Geometry: final body of the model. Coordinates: model frame, mm. Round coordinates to 2 decimals unless told otherwise and drop trailing zeros. Order: outer loops, then holes, each group sorted by start corner. A loop starts at its lowest first (then second) coordinate and runs counter-clockwise, first axis right, second up. Notation, with made-up numbers: M 70,44.5 L 112,44.5 A30 cw 112,72.5 Z; hole C 82.25,38 d10. An arc over 180 degrees is marked long. Return JSON: item names as keys, results as strings. Group by question number.
Q1. Contact query for flat-ended pins moving along their axis: pin 1 (5 mm diameter, centred on x = -5, y = -8, fed in from +Z); pin 2 (10 mm diameter, centred on x = 0, z = -6, fed in from -Y); pin 3 (1.1 mm diameter, centred on y = 3, z = 59, fed in from +X). Output: stop coordinate, or through.
Q2. Cut plane A-A on x = 5. Output: boundary loops of the cut face in (y, z), and give its area (3 significant figures).
Q3. Cut plane C-C on z = -23.5. Output: boundary loops of the cut face in (x, y).
Q4. Ray query, probe 1 along Y at (x, z) = (3.5, -9); probe 2 along Z at (x, y) = (8, -3); probe 3 along Z at (x, y) = (-9.5, 3). Return the intervals inside material, ascending.
Q5. Cut plane B-B on y = -7.5. Output: boundary loops of the cut face in (x, z).
```python
from build123d import *

# Parameters (mm, degrees)
SKETCH1_W           = 36
SKETCH1_H           = 1
BOSS_EXTRUDE1_DEPTH = 65
BOSS_EXTRUDE2_DEPTH = 5
SKETCH3_W           = 36
SKETCH3_H           = 2
BOSS_EXTRUDE3_DEPTH = 10
CUT_EXTRUDE1_REACH  = 76.334


with BuildPart() as part:
    # Sketch1 → Boss-Extrude1 (new, symmetric)
    with BuildSketch(Plane.XY):
        Rectangle(SKETCH1_W, SKETCH1_H)
    extrude(amount=BOSS_EXTRUDE1_DEPTH, both=True)

    # Sketch2 → Boss-Extrude2 (add, symmetric)
    with BuildSketch(Plane.XY.offset(60)):
        Polygon((-15, 0.5), (-15, 2.5), (-16.5, 2.5), (-16.5, 3.5), (16.5, 3.5), (16.5, 2.5), (15, 2.5), (15, 0.5), align=None)
    extrude(amount=BOSS_EXTRUDE2_DEPTH, both=True)

    # Sketch3 → Boss-Extrude3 (add)
    with BuildSketch(Plane.XZ.offset(0.5)):
        with Locations((0, -54)):
            Rectangle(SKETCH3_W, SKETCH3_H)
    extrude(amount=BOSS_EXTRUDE3_DEPTH)

    # Sketch4 → Cut-Extrude1 (cut, up to next)
    with BuildSketch(Plane(origin=(16.5, 0, 0), x_dir=(0, 0, -1), z_dir=(1, 0, 0)), mode=Mode.PRIVATE) as cut_extrude1_sk1:
        Polygon((-57, 3.5), (-55, 2.5), (-55, 3.5), align=None)
    cut_extrude1_tool1 = extrude(cut_extrude1_sk1.sketch, amount=-CUT_EXTRUDE1_REACH, mode=Mode.PRIVATE) & part.part
    add(cut_extrude1_tool1.solids().sort_by_distance((16.5, 3.166667, 55.666667))[0], mode=Mode.SUBTRACT)


solid = part.part
```
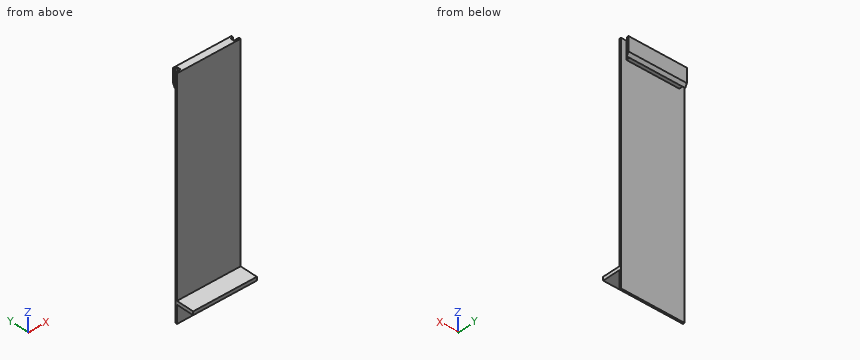
Result sheet:
{
 "1": {"pin 1": "stops at z = -53", "pin 2": "stops at y = -0.5", "pin 3": "stops at x = 16.5"},
 "2": {"outline": "M -10.5,-55 L -0.5,-55 L -0.5,-65 L 0.5,-65 L 0.5,55 L 2.5,55 L 3.5,57 L 3.5,65 L -0.5,65 L -0.5,-53 L -10.5,-53 Z", "area": "179 mm²"},
 "3": {"outline": "M -18,-0.5 L 18,-0.5 L 18,0.5 L -18,0.5 Z"},
 "4": {"probe 1": "y = -0.5 to 0.5", "probe 2": "z = -55 to -53", "probe 3": "z = 56 to 65"},
 "5": {"outline": "M -18,-55 L 18,-55 L 18,-53 L -18,-53 Z"}
}
